Verification items for the finished model (mm, model axes). A direction names the side the tool comes from. Coordinates: 2 decimals unless noted, no trailing zeros. Loops run counter-clockwise (first coordinate to the right, second up) from the corner with the lowest first, then second, coordinate; pieces in that order, holes last. Notation, with made-up numbers: (76, 39.25) - (87, 39.25) arc R29 ccw to (87, 64.25) - close; hole circle Ø8 at (-7, 48.5). An arc over 180 degrees is marked (long way). One line per item, written item: value. Start each with the question number.
(1) Gauge pin test, flat ends, axial feed: P1, Ø1.5, axis at y = -26.5, z = 26, coming from the +X side; P2, Ø8, axis at x = 18, z = 11.5, coming from the -Y side; P3, Ø12, axis at x = 19.5, y = -33.5, coming from the +Z side. Record the tip position at first contact, or that the pin passes through.
(2) Set-up check for faces 1 (the face through (19, -12.07, 16)), 2 (the face through (25.58, -28.07, 15.55)): record each of +Z, -Z, +X, -X, +Y, -Y from which the full face is reachable in a straight line by a thin tool's end or side.
(3) Section check B-B (y = -31.75). Record the boundary of the cut face in (x, z), plus the area to 3 significant figures.
(4) Thickness scan on probe 1 along X at (y, z) = (-28, 25); probe 2 along Z at (x, y) = (31, -18.5); probe 3 along Y at (x, z) = (15, 21). Record the ranges inside material, lowest first. Write a range as [from, to].
(5) Section check A-A (z = 6). Record the boundary of the cut face in (x, y).
(6) Section check C-C (x = 19). Record the boundary of the cut face in (y, z), plus the area to 3 significant figures.
```python
from build123d import *

# Parameters (mm, degrees)
F0_W     = 25.6966426969
F0_H     = 31.5367914736
F1_DEPTH = 38.1
F3_DEPTH = 25.4
F4_DEPTH = 50.8


with BuildPart() as f1:
    # F0 (on Right) → F1 (new body)
    with BuildSketch(Plane.YZ):
        with Locations((-24.9179564416, 15.7683957368)):
            Rectangle(F0_W, F0_H)
    extrude(amount=F1_DEPTH)

    # F2 (on face) → F3 (join)
    with BuildSketch(Plane.YZ.offset(38.1)):
        Polygon((-37.7662777901, 0), (-18.1044526398, 31.5367914736), (-37.7662777901, 31.5367914736), align=None)
    extrude(amount=F3_DEPTH)

    # F4 (cut): a face of the model
    f4_faces = [f1.faces().sort_by_distance(p)[0] for p in [
        (63.5, -31.2123360733, 21.0245276491),
    ]]
    extrude(f4_faces, amount=-F4_DEPTH, mode=Mode.SUBTRACT)


solid = f1.part
```
Responses:
1. P1: stops at x = 12.7
1. P2: stops at y = -33.09
1. P3: stops at z = 16.47
2. face 1: +Z, -Z, +X, -X, +Y
2. face 2: +Z, +X, -Y
3. outline: (0, 0) - (38.1, 0) - (38.1, 9.65) - (12.7, 9.65) - (12.7, 31.54) - (0, 31.54) - close
3. area: 646 mm²
4. probe 1: x = [0, 12.7]
4. probe 2: z = [0, 30.9]
4. probe 3: y = [-24.67, -12.07]
5. outline: (0, -37.77) - (12.7, -37.77) - (12.7, -34.03) - (38.1, -34.03) - (38.1, -12.07) - (0, -12.07) - close
6. outline: (-37.77, 0) - (-12.07, 0) - (-12.07, 31.54) - (-18.1, 31.54) - close
6. area: 500 mm²
